Could you check a few things on this model? Use its own coordinates, in mm. Round coordinates to 2 decimals unless told otherwise and drop trailing zeros. Write each loop counter-clockwise with the first axis right and the second up, starting at its lowest first coordinate (ties: lowest second). Pieces come first, ordered by that corner, then holes. Notation, with made-up numbers: (12.25, -13.5) -> (29.25, -13.5) arc R5 cw to (29.25, -8.5) -> close; hole circle Ø6 at (-38, 71.25). An arc over 180 degrees is marked (long way). Answer in a Markdown table with one row per item.
from build123d import *

# Parameters (mm, degrees)
SKETCH1_W           = 609.6
SKETCH1_H           = 152.4
BOSS_EXTRUDE1_DEPTH = 3.175
SKETCH2_R           = 2.875
SKETCH2_R_2         = 2
CUT_EXTRUDE1_DEPTH  = 341.835917268


with BuildPart() as part:
    # Sketch1 → Boss-Extrude1 (new, symmetric)
    with BuildSketch(Plane(origin=(0, 0, 0), x_dir=(1, 0, 0), z_dir=(0, 1, 0))):
        with Locations((0, -76.2)):
            Rectangle(SKETCH1_W, SKETCH1_H)
    boss_extrude1 = extrude(amount=BOSS_EXTRUDE1_DEPTH, both=True)

    # Sketch2 → Cut-Extrude1 (cut, through all)
    with BuildSketch(Plane(origin=(0, -3.175, 0), x_dir=(1, 0, 0), z_dir=(0, 1, 0))):
        Polygon((34.71, -136.45), (34.71, -139.65), (36.1, -139.65), (36.1, -146.05), (0, -146.05), (0, -152.4), (76.2, -152.4), (76.2, -146.05), (40.1, -146.05), (40.1, -139.65), (41.49, -139.65), (41.49, -136.45), (40.1, -136.45), (40.1, -127.4), (36.1, -127.4), (36.1, -136.45), align=None)
        Polygon((-304.8, -146.05), (-304.8, -152.4), (-228.6, -152.4), (-228.6, -146.05), (-264.7, -146.05), (-264.7, -139.65), (-263.31, -139.65), (-263.31, -136.45), (-264.7, -136.45), (-264.7, -127.4), (-268.7, -127.4), (-268.7, -136.45), (-270.09, -136.45), (-270.09, -139.65), (-268.7, -139.65), (-268.7, -146.05), align=None)
        Polygon((-152.4, -146.05), (-152.4, -152.4), (-76.2, -152.4), (-76.2, -146.05), (-112.3, -146.05), (-112.3, -139.65), (-110.91, -139.65), (-110.91, -136.45), (-112.3, -136.45), (-112.3, -127.4), (-116.3, -127.4), (-116.3, -136.45), (-117.69, -136.45), (-117.69, -139.65), (-116.3, -139.65), (-116.3, -146.05), align=None)
        Polygon((152.4, -146.05), (152.4, -152.4), (228.6, -152.4), (228.6, -146.05), (192.5, -146.05), (192.5, -139.65), (193.89, -139.65), (193.89, -136.45), (192.5, -136.45), (192.5, -127.4), (188.5, -127.4), (188.5, -136.45), (187.11, -136.45), (187.11, -139.65), (188.5, -139.65), (188.5, -146.05), align=None)
        with Locations(Location((289.39, -138.999999876, 0), (0, 0, 90))):
            Circle(SKETCH2_R)
        with Locations(Location((259.53, -138.999999876, 0), (0, 0, 90))):
            Circle(SKETCH2_R)
        with Locations(Location((266.7, -149.225, 0), (0, 0, 90))):
            Circle(SKETCH2_R_2)
        with Locations(Location((114.3, -149.225, 0), (0, 0, 90))):
            Circle(SKETCH2_R_2)
        with Locations(Location((-38.1, -149.225, 0), (0, 0, 90))):
            Circle(SKETCH2_R_2)
        with Locations(Location((-190.5, -149.225, 0), (0, 0, 90))):
            Circle(SKETCH2_R_2)
    cut_extrude1 = extrude(amount=CUT_EXTRUDE1_DEPTH, mode=Mode.SUBTRACT)

    # Mirror1: Boss-Extrude1, Cut-Extrude1 across plane
    add(boss_extrude1.mirror(Plane(origin=(0, 3.175, 0), x_dir=(1, 0, 0), z_dir=(0, 0, 1))))
    add(cut_extrude1.mirror(Plane(origin=(0, 3.175, 0), x_dir=(1, 0, 0), z_dir=(0, 0, 1))), mode=Mode.SUBTRACT)


solid = part.part
1) Imagine slicing it at A-A, the plane y = 0.5. Count the separate pieces of the cut face and the enclosed holes in it, plus the area to 3 significant figures.
Findings:
| item | result |
|---|---|
| separate pieces | 1 |
| enclosed holes | 12 |
| area | 181,000 mm^2 |
2) Please list where these lines run through material, in increasing order: line 1 (Z direction, x = 259.53, y = 0.75) (3 decimals); line 2 (X direction, y = -1.5, z = -133); line 3 (Z direction, x = -147.5, y = 1.75).
Findings:
| item | result |
|---|---|
| line 1 | z = -152.4 to -141.875, -136.125 to 136.125, 141.875 to 152.4 |
| line 2 | x = -304.8 to -268.7, -264.7 to -116.3, -112.3 to 36.1, 40.1 to 188.5, 192.5 to 304.8 |
| line 3 | z = -146.05 to 146.05 |
3) For pin 1 (2 mm diameter, centred on x = -267, y = 0.5, fed in from +Z); pin 2 (2 mm diameter, centred on x = 190, y = 0.5, fed in from -Z); pin 3 (1.5 mm diameter, centred on x = -117, y = 0, fed in from -Z), each with a flat end and sliding along its axis, tell me the tip position at first contact or that it passes through.
Findings:
| item | result |
|---|---|
| pin 1 | stops at z = 127.4 |
| pin 2 | stops at z = -127.4 |
| pin 3 | stops at z = -146.05 |
4) Imagine slicing it at B-B, the plane x = 167. Please give me the cut outline in (y, z) (3 decimals).
Findings:
| item | result |
|---|---|
| outline | (-3.175, -146.05) -> (3.175, -146.05) -> (3.175, 146.05) -> (-3.175, 146.05) -> close |
